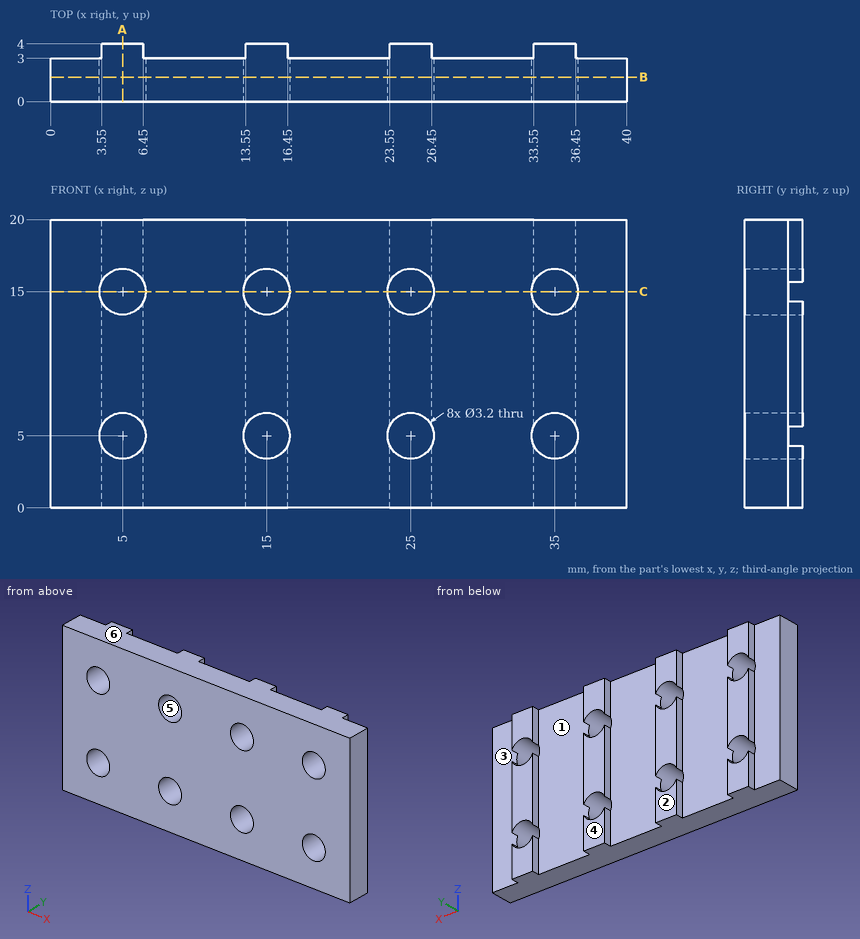
Verification items for this drawing (mm, ordinates from the low corner). A direction names the side the tool comes from. Give positions to 0.01 mm unless a question says otherwise; leave off trailing zeros. Write each loop counter-clockwise with the first axis right and the second up, starting at its lowest first coordinate (ties: lowest second). Pieces come first, ordered by that corner, then holes. Notation, with made-up numbers: M 85.25,74 L 93.25,74 A19 ccw 93.25,107 Z; hole C 4.25,-11.5 d11. An arc over 180 degrees is marked long. Use one line per item in the form item = value.
(1) Section check C-C on z = 15. Record the boundary of the cut face in (x, y).
Answer block:
outline = M 0,0 L 3.4,0 L 3.4,3 L 0,3 Z; M 6.6,0 L 13.4,0 L 13.4,3 L 6.6,3 Z; M 16.6,0 L 23.4,0 L 23.4,3 L 16.6,3 Z; M 26.6,0 L 33.4,0 L 33.4,3 L 26.6,3 Z; M 36.6,0 L 40,0 L 40,3 L 36.6,3 Z
(2) Draft check along Z on the marked faces 4, 5 and 6. Enter one of: pulls with the +Z half, pulls with the -Z half, needs draft (parallel to the pull), parting line crosses it, or undercut.
Answer block:
face_4 = needs draft
face_5 = undercut
face_6 = pulls with the +Z half
(3) Material ranges on line 1 along Z through (x, y) = (35, 1.3); line 2 along X through (y, z) = (2.4, 15); line 3 along X through (y, z) = (3.5, 7), recorded low to high.
Answer block:
line_1 = 0 to 3.4, 6.6 to 13.4, 16.6 to 20
line_2 = 0 to 3.4, 6.6 to 13.4, 16.6 to 23.4, 26.6 to 33.4, 36.6 to 40
line_3 = 3.55 to 6.45, 13.55 to 16.45, 23.55 to 26.45, 33.55 to 36.45
(4) Tool access check on the marked faces 1, 2 and 3. Record the directions out of +Z, -Z, +X, -X, +Y, -Y that give a thin tool (end or side, any length) a straight path to the whole face; none if there is none.
Answer block:
face_1 = +Z, -Z, +Y
face_2 = +Z, -Z, +X, -X, +Y
face_3 = +Z, -Z, +X, +Y
(5) Depth check by flat-ended pin: P1, Ø2, axis at x = 18.5, z = 13, coming from the +Y side; P2, Ø1.5, axis at x = 5, z = 7.5, coming from the -Y side; P3, Ø0.8, axis at y = 3.5, z = 18, coming from the +X side. Enter the tip coordinate at first touch or a pass-through.
Answer block:
P1 = 3
P2 = 0
P3 = 36.45
(6) Section check B-B on y = 1.7. State how many separate pieces and enclosed holes the cut face has, plus the area to 3 significant figures.
Answer block:
separate_pieces = 1
enclosed_holes = 8
area = 736 mm2
(7) Section check A-A on x = 5. Record the boundary of the cut face in (y, z).
Answer block:
outline = M 0,0 L 4,0 L 4,3.4 L 0,3.4 Z; M 0,6.6 L 4,6.6 L 4,13.4 L 0,13.4 Z; M 0,16.6 L 4,16.6 L 4,20 L 0,20 Z
